The model under review builds one solid part; all positions refer to its coordinate system, in mm. Face numbers are marked on the shaded views. A direction names the side the tool comes from. Coordinates: 2 decimals unless noted, no trailing zeros. Order: outer loops, then holes, each group sorted by start corner. A loop starts at its lowest first (then second) coordinate and runs counter-clockwise, first axis right, second up.
from build123d import *

# Parameters (mm, degrees)
BOSS_EXTRUDE1_DEPTH = 37.5
SKETCH3_R           = 1.8
CUT_EXTRUDE1_DEPTH  = 40.623984608
CUT_EXTRUDE2_DEPTH  = 40.623984608


with BuildPart() as part:
    # Sketch2 → Boss-Extrude1 (new, symmetric)
    with BuildSketch(Plane.XY):
        with BuildLine():
            Line((-6.35, -6.35), (6.35, -6.35))
            Line((6.35, -6.35), (6.35, 6.35))
            Line((6.35, 6.35), (5.55625, 6.35))
            ThreePointArc((5.55625, 6.35), (4.994983992, 6.117516008), (4.7625, 5.55625))
            Line((4.7625, 5.55625), (4.7625, -3.1877))
            ThreePointArc((4.7625, -3.1877), (4.301251759, -4.301251759), (3.1877, -4.7625))
            Line((3.1877, -4.7625), (-5.55625, -4.7625))
            ThreePointArc((-5.55625, -4.7625), (-6.117516008, -4.994983992), (-6.35, -5.55625))
            Line((-6.35, -5.55625), (-6.35, -6.35))
        make_face()
    extrude(amount=BOSS_EXTRUDE1_DEPTH, both=True)

    # Sketch3 → Cut-Extrude1 (cut, through all)
    with BuildSketch(Plane(origin=(0, -4.7625, 0), x_dir=(1, 0, 0), z_dir=(0, 1, 0))):
        with Locations(Location((-1.0623, 25, 0), (0, 0, 180))):
            Circle(SKETCH3_R)
        with Locations(Location((-1.0623, -25, 0), (0, 0, 180))):
            Circle(SKETCH3_R)
        with Locations(Location((-1.0623, 0, 0), (0, 0, 180))):
            Circle(SKETCH3_R)
    extrude(amount=-CUT_EXTRUDE1_DEPTH, mode=Mode.SUBTRACT)

    # Sketch4 → Cut-Extrude2 (cut, through all)
    with BuildSketch(Plane.ZY.offset(-4.7625)):
        with BuildLine():
            Line((-32.7, 2.85625), (32.7, 2.85625))
            ThreePointArc((32.7, 2.85625), (33.548528137, 2.504778137), (33.9, 1.65625))
            Line((33.9, 1.65625), (33.9, 0.45625))
            ThreePointArc((33.9, 0.45625), (33.548528137, -0.392278137), (32.7, -0.74375))
            Line((32.7, -0.74375), (-32.7, -0.74375))
            ThreePointArc((-32.7, -0.74375), (-33.548528137, -0.392278137), (-33.9, 0.45625))
            Line((-33.9, 0.45625), (-33.9, 1.65625))
            ThreePointArc((-33.9, 1.65625), (-33.548528137, 2.504778137), (-32.7, 2.85625))
        make_face()
    extrude(amount=-CUT_EXTRUDE2_DEPTH, mode=Mode.SUBTRACT)


solid = part.part
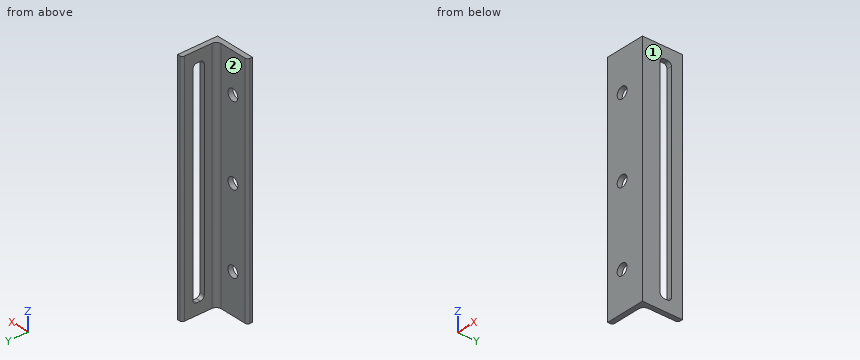
(1) Consider section A-A (z = -25). Give the boundary of the cut face in (x, y), then the cut area to 3 significant figures.
(2) Consider section B-B (z = 3). Give the boundary of the cut face in (x, y).
(3) Insertion check: pin 1 Ø2.5 at (x, z) = (-2, 11) entering from +Y; pin 2 Ø3 at (x, y) = (3, 1) entering from +Z. Each pin has a flat end and moves straight along its axis. Give the tip position at first contact, or say it passes through.
(4) Wall thickness on line 1 (Y direction, x = -4.5, z = -16); line 2 (Y direction, x = 5.75, z = 20); line 3 (X direction, y = -1, z = 11.5): over which ranges is each line inside the solid? List them lowest first.
(5) Tool access review of the marked faces 1 and 2: name each direction out of +Z, -Z, +X, -X, +Y, -Y from which nothing blocks a thin tool from reaching the whole face with its end or side.
Findings:
1. outline: (-6.35, -6.35) - (-2.86, -6.35) - (-2.86, -4.76) - (-5.56, -4.76) arc R0.79 ccw to (-6.35, -5.56) - close; (0.74, -6.35) - (6.35, -6.35) - (6.35, -0.74) - (4.76, -0.74) - (4.76, -3.19) arc R1.57 cw to (3.19, -4.76) - (0.74, -4.76) - close; (4.76, 2.86) - (6.35, 2.86) - (6.35, 6.35) - (5.56, 6.35) arc R0.79 ccw to (4.76, 5.56) - close
1. area: 26.6 mm2
2. outline: (-6.35, -6.35) - (6.35, -6.35) - (6.35, -0.74) - (4.76, -0.74) - (4.76, -3.19) arc R1.57 cw to (3.19, -4.76) - (-5.56, -4.76) arc R0.79 ccw to (-6.35, -5.56) - close; (4.76, 2.86) - (6.35, 2.86) - (6.35, 6.35) - (5.56, 6.35) arc R0.79 ccw to (4.76, 5.56) - close
3. pin 1: stops at y = -4.76
3. pin 2: passes through
4. line 1: y = -6.35 to -4.76
4. line 2: y = -6.35 to -0.74, 2.86 to 6.35
4. line 3: x = 4.76 to 6.35
5. face 1: +Z, -Z, +X, +Y, -Y
5. face 2: +Z, -Z, -X, +Y
